Source: CAD feature listing. Evaluate the final solid. Frame: model axes, mm. Give positions to 0.01 mm unless a question says otherwise; leave off trailing zeros. Write each loop counter-clockwise with the first axis right and the second up, starting at its lowest first coordinate (ties: lowest second). Pieces come first, ordered by that corner, then holes. Notation, with made-up numbers: (40, -3) -> (82, -3) arc R27 ccw to (82, 27) -> close; hole circle Ø5 at (12.5, -13.5). An arc over 180 degrees is marked (long way). Answer as a JSON object with one key per item and string values. Group by question number.
Item 1: Ray query, probe 1 along X at (y, z) = (2, -2); probe 2 along X at (y, z) = (1, -1); probe 3 along Z at (x, y) = (-1.25, 5.5). Return the intervals inside material, ascending. Write a range as from..to.
Item 2: Section query C-C on z = -1.25. Return the cut outline in (x, y), plus the area to 3 significant figures.
Item 3: Section query A-A on z = 1.5. Return the cut outline in (x, y), plus the area to 3 significant figures.
Item 4: First-contact query: pin 1 Ø0.6 at (x, y) = (1.5, -0.5) entering from -Z; pin 2 Ø1 at (x, y) = (-1, -2.5) entering from -Z; pin 3 Ø1.4 at (x, y) = (1, -0.5) entering from +Z; pin 4 Ø8 at (y, z) = (-1.5, -2) entering from +X. Flat tips, straight axial feed; report the tip coordinate or a pass-through.
Item 5: Section query D-D on x = -0.75. Return the cut outline in (y, z).
Item 6: Section query B-B on y = 1.75. Return the cut outline in (x, z), plus the area to 3 significant figures.
from build123d import *

# Parameters (mm, degrees)
F3_W     = 1.248711
F3_H     = 5.586524
F4_DEPTH = 25.4


with BuildPart() as f1:
    # F0 (on Front) → F1 (revolve)
    with BuildSketch(Plane.XZ):
        with BuildLine():
            Line((-7.62, 0), (7.62, 0))
            ThreePointArc((7.62, 0), (0, 7.62), (-7.62, 0))
        make_face()
    revolve(axis=Axis((0, 0, 0), (1, 0, 0)))

    # F3 (on offset) → F4 (cut)
    with BuildSketch(Plane.XZ.offset(8.89)):
        with Locations((-1.070891, 0)):
            Rectangle(F3_W, F3_H)
        with Locations((1.070891, 0)):
            Rectangle(F3_W, F3_H)
    extrude(amount=-F4_DEPTH, mode=Mode.SUBTRACT)


solid = f1.part
Worked answers:
{
 "1": {"probe 1": "-7.08..-1.7, -0.45..0.45, 1.7..7.08", "probe 2": "-7.49..-1.7, -0.45..0.45, 1.7..7.49", "probe 3": "-5.12..-2.79, 2.79..5.12"},
 "2": {"outline": "(-1.7, -7.32) -> (-1.7, 7.32) arc R7.52 ccw to start; (-0.45, -7.5) arc R7.52 ccw to (0.45, -7.5) -> (0.45, 7.5) arc R7.52 ccw to (-0.45, 7.5) -> close; (1.7, -7.32) arc R7.52 ccw to (1.7, 7.32) -> close", "area": "140 mm^2"},
 "3": {"outline": "(-1.7, -7.28) -> (-1.7, 7.28) arc R7.47 ccw to start; (-0.45, -7.46) arc R7.47 ccw to (0.45, -7.46) -> (0.45, 7.46) arc R7.47 ccw to (-0.45, 7.46) -> close; (1.7, -7.28) arc R7.47 ccw to (1.7, 7.28) -> close", "area": "138 mm^2"},
 "4": {"pin 1": "z = -7.51", "pin 2": "z = -7.3", "pin 3": "z = 7.61", "pin 4": "x = 7.62"},
 "5": {"outline": "(-7.05, -2.79) arc R7.58 ccw to (7.05, -2.79) -> close; (-7.05, 2.79) -> (7.05, 2.79) arc R7.58 ccw to start"},
 "6": {"outline": "circle Ø14.83 at (0, 0); hole (-1.7, -2.79) -> (-0.45, -2.79) -> (-0.45, 2.79) -> (-1.7, 2.79) -> close; hole (0.45, -2.79) -> (1.7, -2.79) -> (1.7, 2.79) -> (0.45, 2.79) -> close", "area": "159 mm^2"}
}
